For this review, take the finished solid that the model builds, in its own axes (mm). A direction names the side the tool comes from. Coordinates: 2 decimals unless noted, no trailing zeros. Order: outer loops, then holes, each group sorted by start corner. A loop starts at its lowest first (then second) coordinate and runs counter-clockwise, first axis right, second up. Notation, with made-up numbers: (38.5, 71) -> (50.5, 71) arc R30 cw to (50.5, 102) -> close; hole circle Ø3 at (-8, 74). An arc over 180 degrees is marked (long way). Write item = value, one per line. Start each with the question number.
1) Consider section C-C on x = 897. Give the boundary of the cut face in (y, z).
2) Insertion check: pin 1 Ø1.5 at (x, y) = (829.5, 541.5) entering from +Z; pin 2 Ø3 at (x, y) = (886, 503) entering from -Z. Each pin has a flat end and moves straight along its axis. Give the tip position at first contact, or say it passes through.
3) Machinability: for faces 4 (the face through (910, 514, -101)), 5 (the face through (836, 516, 0)), which of the approach directions +Z, -Z, +X, -X, +Y, -Y give a long, thin tool a straight path to every point of the face, cutting with its end or side? Answer none if there is none.
4) Draft analysis for pull direction Y (two halves, no side actions). For faces 1 (the face through (836, 585, -96)), 2 (the face through (836, 469, -190)), 3 (the face through (839, 475, -101)), state which applies: +Y half, -Y half, draft (parallel to the pull), parting line (faces both ways), or undercut.
5) Wall thickness on probe 1 along Y at (x, z) = (835, -174); probe 2 along X at (y, z) = (514, -63); probe 3 along Z at (x, y) = (834.5, 532): over which ranges is each line inside the solid? List them lowest first. Write a range as [from, to].
6) Consider section B-B on y = 548.5. Give the boundary of the cut face in (x, z).
7) Consider section A-A on z = -64. Give the boundary of the cut face in (x, y).
from build123d import *

# Parameters (mm, degrees)
BOX124_W     = 140
BOX124_H     = 80
BOX124_DEPTH = 190
BOX123_W     = 140
BOX123_H     = 80
BOX123_DEPTH = 180
BOX122_W     = 195
BOX122_H     = 140
BOX122_DEPTH = 190


with BuildPart() as cube096:
    # Box124 → Box124 (new body)
    with BuildSketch(Plane(origin=(220, 30, 0), x_dir=(1, 0, 0), z_dir=(0, 0, 1))):
        with Locations((70, 40)):
            Rectangle(BOX124_W, BOX124_H)
    extrude(amount=BOX124_DEPTH)


with BuildPart() as fusion024:
    # Box123 → Box123 (new body)
    with BuildSketch(Plane(origin=(30, 30, 0), x_dir=(1, 0, 0), z_dir=(0, 0, 1))):
        with Locations((70, 40)):
            Rectangle(BOX123_W, BOX123_H)
    extrude(amount=BOX123_DEPTH)

    # Fusion024: union Cube096
    add(cube096.part)


with BuildPart() as obj1:
    # Box122 → Box122 (new body)
    with BuildSketch(Plane.XY):
        with Locations((97.5, 70)):
            Rectangle(BOX122_W, BOX122_H)
    extrude(amount=BOX122_DEPTH)

    # Cut019: cut Fusion024
    add(fusion024.part, mode=Mode.SUBTRACT)


with BuildPart() as obj1_1:
    # Cut019 placement: moved
    add(obj1.part.moved(Location((740, 445, -190))))


solid = obj1_1.part
Answer sheet:
q1.outline = (445, -190) -> (475, -190) -> (475, -10) -> (555, -10) -> (555, -190) -> (585, -190) -> (585, 0) -> (445, 0) -> close
q2.pin_1 = 0
q2.pin_2 = -10
q3.face_4 = -Z
q3.face_5 = +Z, +X, -X, +Y, -Y
q4.face_1 = +Y half
q4.face_2 = draft
q4.face_3 = undercut
q5.probe_1 = [445, 475], [555, 585]
q5.probe_2 = [740, 770], [910, 935]
q5.probe_3 = [-10, 0]
q6.outline = (740, -190) -> (770, -190) -> (770, -10) -> (910, -10) -> (910, -190) -> (935, -190) -> (935, 0) -> (740, 0) -> close
q7.outline = (740, 445) -> (935, 445) -> (935, 585) -> (740, 585) -> close; hole (770, 475) -> (910, 475) -> (910, 555) -> (770, 555) -> close
